Here's how the part is built. I have some questions about the finished solid (model axes, mm). A direction names the side the tool comes from. Give positions to 0.01 mm unless a question says otherwise; leave off trailing zeros. Loops run counter-clockwise (first coordinate to the right, second up) from the corner with the lowest first, then second, coordinate; pieces in that order, holes last.
Q1. Thinking about a two-plate mould opening in X: for faces 1 (the face through (43.61, 13.73, 2.63)), 2 (the face through (40.43, -13.33, 5.334)), 3 (the face through (-30.235, -23.183, 7.012)), which applies, pulls with the +X half, pulls with the -X half, needs draft (parallel to the pull), parting line crosses it, or undercut?
Q2. Suppose I cut it at A-A (x = 0). List the corners of the cut face in (y, z) for me.
Q3. I'm going to push flat-ended pins straight in: P1, Ø2, axis at x = -5.5, z = 5.5, coming from the -Y side; P2, Ø4, axis at y = 28.5, z = 2, coming from the -X side; P3, Ø1, axis at y = 14.5, z = 6.5, coming from the +X side. Where does each tip first touch, or does it pass through?
Q4. For faces 4 (the face through (-1, 1, 5.08)), 5 (the face through (-35, 16, 8.89)), which set-ups out of +Z, -Z, +X, -X, +Y, -Y let a thin tool reach every point of the face, with its end or its side?
Q5. Suppose I cut it at C-C (z = 3.5). List the corners of the cut face in (x, y) for me.
Q6. I need wall thicknesses on probe 1 along Y at (x, z) = (0, 7.6); probe 2 along Z at (x, y) = (-14.5, -3); probe 3 along Y at (x, z) = (-2, 6.25). Which ranges of each line are inside material? Lowest first, please.
```python
from build123d import *

# Parameters (mm, degrees)
F0_R     = 45.72
F1_DEPTH = 5.334
F2_R     = 42.418
F3_DEPTH = 8.89
F4_R     = 38.1
F5_DEPTH = 3.81


with BuildPart() as f1:
    # F0 (on Top) → F1 (new body)
    with BuildSketch(Plane.XY):
        Circle(F0_R)
    extrude(amount=F1_DEPTH)

    # F2 (on Top) → F3 (join)
    with BuildSketch(Plane.XY):
        Circle(F2_R)
    extrude(amount=F3_DEPTH)

    # F4 (on face) → F5 (cut)
    with BuildSketch(Plane.XY.offset(8.89)):
        Circle(F4_R)
    extrude(amount=-F5_DEPTH, mode=Mode.SUBTRACT)


solid = f1.part
```
Solutions:
1. face 1: parting line crosses it
1. face 2: needs draft
1. face 3: undercut
2. outline: (-45.72, 0) - (45.72, 0) - (45.72, 5.33) - (42.42, 5.33) - (42.42, 8.89) - (38.1, 8.89) - (38.1, 5.08) - (-38.1, 5.08) - (-38.1, 8.89) - (-42.42, 8.89) - (-42.42, 5.33) - (-45.72, 5.33) - close
3. P1: stops at y = -45.5
3. P2: stops at x = -37.26
3. P3: stops at x = 40.04
4. face 4: +Z
4. face 5: +Z, +X, -X, +Y, -Y
5. outline: circle Ø91.44 at (0, 0)
6. probe 1: y = -42.42 to -38.1, 38.1 to 42.42
6. probe 2: z = 0 to 5.08
6. probe 3: y = -42.37 to -38.05, 38.05 to 42.37
